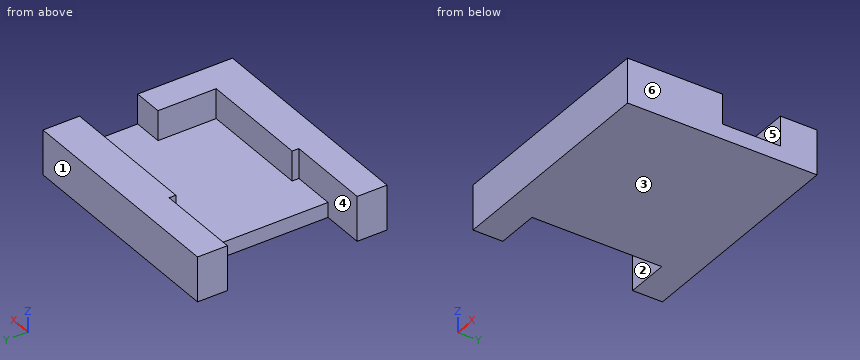
from build123d import *

# Parameters (mm, degrees)
F0_W      = 19.05
F0_H      = 19.812
F1_DEPTH  = 2.54
F2_DEPTH  = 2.54
F0_W_2    = 14.605
F0_H_2    = 1.143
F3_DEPTH  = 2.54
F4_W      = 38.735
F4_H      = 32.258
F5_DEPTH  = 7.62
F6_DEPTH  = 7.62
F7_W      = 7.3025
F7_H      = 22.098
F8_DEPTH  = 2.54
F9_W      = 5.08
F9_H      = 9.906
F10_DEPTH = 5.08


with BuildPart() as f1:
    # F0 (on Top) → F1 (new body)
    with BuildSketch(Plane.XY):
        with Locations((9.525, 9.906)):
            Rectangle(F0_W, F0_H)
    extrude(amount=F1_DEPTH)

    # F0 (on Top) → F2 (join)
    with BuildSketch(Plane.XY):
        Polygon((-14.605, 0), (0, 0), (0, 19.812), (0, 20.955), (-14.605, 20.955), align=None)
    extrude(amount=F2_DEPTH)

    # F0 (on Top) → F3 (join)
    with BuildSketch(Plane.XY):
        with Locations((-7.3025, -0.5715)):
            Rectangle(F0_W_2, F0_H_2)
    extrude(amount=F3_DEPTH)

    # F4 (on Top) → F5 (join)
    with BuildSketch(Plane.XY):
        with Locations((4.7625, 9.906)):
            Rectangle(F4_W, F4_H)
    extrude(amount=-F5_DEPTH)

    # F3_face (on face) → F6 (cut)
    with BuildSketch(Plane(origin=(1.768302, 9.906, 2.54), x_dir=(1, 0, 0), z_dir=(0, 0, 1))):
        Polygon((-1.768302, -9.906), (17.281698, -9.906), (17.281698, 9.906), (-1.768302, 9.906), (-1.768302, 11.049), (-16.373302, 11.049), (-16.373302, -11.049), (-1.768302, -11.049), align=None)
    extrude(amount=-F6_DEPTH, mode=Mode.SUBTRACT)

    # F7 (on face) → F8 (cut)
    with BuildSketch(Plane.XY.offset(-5.08)):
        with Locations((-10.95375, 9.906)):
            Rectangle(F7_W, F7_H)
    extrude(amount=-F8_DEPTH, mode=Mode.SUBTRACT)

    # F9 (on face) → F10 (cut)
    with BuildSketch(Plane.XY):
        with Locations((21.59, 14.859)):
            Rectangle(F9_W, F9_H)
    extrude(amount=-F10_DEPTH, mode=Mode.SUBTRACT)


solid = f1.part
For this review, take the finished solid that the model builds, in its own axes (mm). Face numbers are marked on the shaded views. A direction names the side the tool comes from. Give positions to 0.01 mm unless a question says otherwise; leave off trailing zeros. Order: outer loops, then holes, each group sorted by start corner. A loop starts at its lowest first (then second) coordinate and runs counter-clockwise, first axis right, second up. Notation, with made-up numbers: M -27,10.5 L 14,10.5 A14 ccw 14,27.5 Z; hole C -22.5,35 d5. An arc over 180 degrees is marked long. Answer in a Markdown table with one row per item. Add a question column.
(1) Wall thickness on probe 1 along Y at (x, z) = (9, -0.25) (3 decimals); probe 2 along Y at (x, z) = (-9, -0.25) (3 decimals); probe 3 along Z at (x, y) = (5, 10): over which ranges is each line inside the solid? List them lowest first. Write a range as [from, to].
(2) Consider section C-C on x = 9.5. State the section outline as (y, z) points (3 decimals).
(3) For pin 1 (11 mm diameter, centred on x = 1, y = 11, fed in from +Z); pin 2 (2.5 mm diameter, centred on y = 5, z = -2, fed in from -X); pin 3 (3 mm diameter, centred on y = 12, z = -7, fed in from -X), all flat-tipped, find the tip position at first contact; note any pin that passes through.
(4) Consider section D-D on z = -5.75. State the section outline as (x, y) points (1 decimal).
(5) Consider section A-A on z = -0.75. State the section outline as (x, y) points (3 decimals), and give its area (3 significant figures).
(6) For the marked faces 4, 5 and 6, list the 3-axis set-ups (+Z, -Z, +X, -X, +Y, -Y) from which the entire face can be reached by the end or side of a thin tool; tool diameter is ignored.
(7) Consider section B-B on x = -10.5. State the section outline as (y, z) points (3 decimals), and give its area (3 significant figures).
(8) Mouldability with a two-part tool opening along Y and no side actions: class the marked faces 1, 2 and 3 as +Y half, -Y half, draft (parallel to the pull), parting line (faces both ways), or undercut.
Evaluation:
| question | item | result |
|---|---|---|
| 1 | probe 1 | y = [-6.223, 0], [19.812, 26.035] |
| 1 | probe 2 | y = [-6.223, -1.143], [20.955, 26.035] |
| 1 | probe 3 | z = [-7.62, -5.08] |
| 2 | outline | M -6.223,-7.62 L 26.035,-7.62 L 26.035,0 L 19.812,0 L 19.812,-5.08 L 0,-5.08 L 0,0 L -6.223,0 Z |
| 3 | pin 1 | stops at z = -5.08 |
| 3 | pin 2 | stops at x = 19.05 |
| 3 | pin 3 | stops at x = -7.3 |
| 4 | outline | M -14.6,-6.2 L 24.1,-6.2 L 24.1,26 L -14.6,26 L -14.6,21 L -7.3,21 L -7.3,-1.1 L -14.6,-1.1 Z |
| 5 | outline | M -14.605,-6.223 L 24.13,-6.223 L 24.13,9.906 L 19.05,9.906 L 19.05,0 L 0,0 L 0,-1.143 L -14.605,-1.143 Z; M -14.605,20.955 L 0,20.955 L 0,19.812 L 24.13,19.812 L 24.13,26.035 L -14.605,26.035 Z |
| 5 | area | 499 mm^2 |
| 6 | face 4 | +Z, -X |
| 6 | face 5 | +Z, +X, -X |
| 6 | face 6 | +Z, -Z, +X, +Y, -Y |
| 7 | outline | M -6.223,-7.62 L -1.143,-7.62 L -1.143,0 L -6.223,0 Z; M 20.955,-7.62 L 26.035,-7.62 L 26.035,0 L 20.955,0 Z |
| 7 | area | 77.4 mm^2 |
| 8 | face 1 | +Y half |
| 8 | face 2 | undercut |
| 8 | face 3 | draft |
